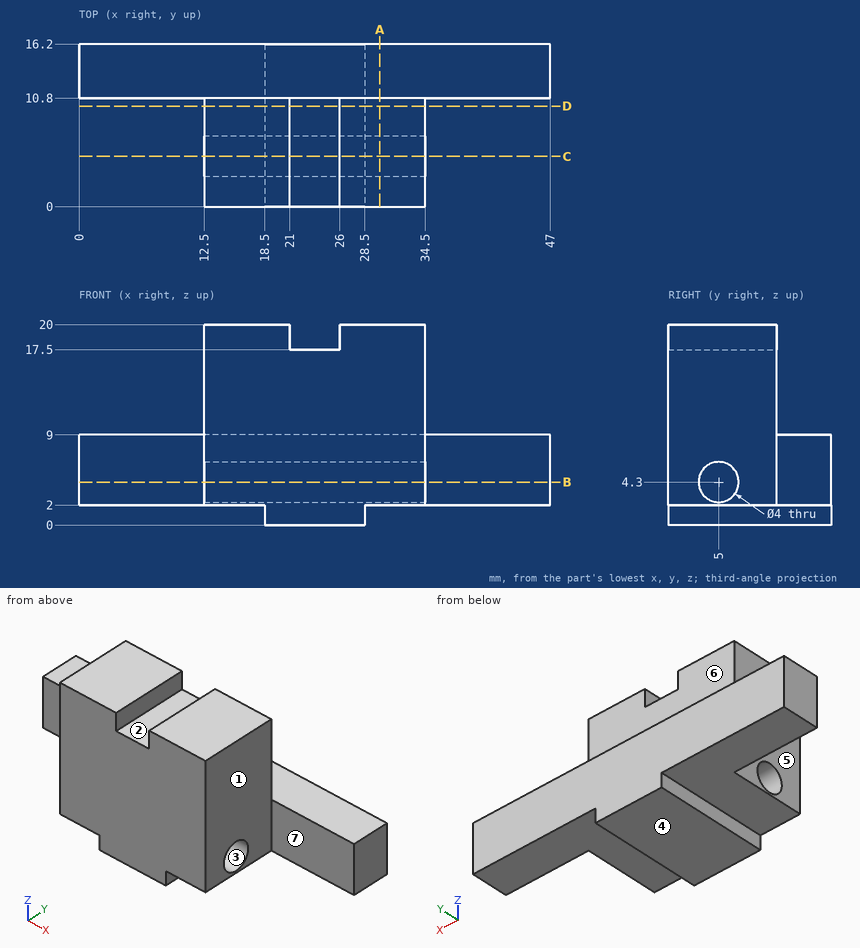
The figure shows three views and two pictorial views of one solid part (mm, origin at its lowest corner). Answer the questions. A direction names the side the tool comes from. Round coordinates to 2 decimals unless told otherwise and drop trailing zeros. Loops run counter-clockwise (first coordinate to the right, second up) from the corner with the lowest first, then second, coordinate; pieces in that order, holes last. Notation, with made-up numbers: M 21,13 L 33,13 A28 cw 33,38 Z; hole C 37.5,-25 d9. An arc over 180 degrees is marked long. Write each question's results on one line, items separated by ' | '. Start each with the question number.
1) Determine the mould class of the marked faces 1, 2, 3 and 4 for opening direction Z: pulls with the +Z half, pulls with the -Z half, needs draft (parallel to the pull), parting line crosses it, or undercut.
2) Find section B-B on z = 4.3. Write down the section's boundary in (x, y).
3) Find section A-A on x = 30. Write down the section's boundary in (y, z).
4) Straight lines are drawn through the part: probe 1 along Z at (x, y) = (28, 5); probe 2 along Z at (x, y) = (17.25, 5); probe 3 along Z at (x, y) = (31.5, 9.5). For each, find the intervals that lie inside material, in ascending order.
5) Find section D-D on y = 10. Write down the section's boundary in (x, z).
6) Which of the six approach directions +Z, -Z, +X, -X, +Y, -Y give full straight-line access (tool end or side, diameter ignored) to the marked faces 5, 6 and 7?
7) Each of these flat-tipped pins is pushed along its axis until it touches: pin 1 (2.5 mm diameter, centred on x = 22.5, y = 5.5, fed in from +Z); pin 2 (6 mm diameter, centred on y = 4.5, z = 5, fed in from +X); pin 3 (5 mm diameter, centred on x = 36, y = 6.5, fed in from -Z). Where does it stop, or does it pass through?
8) Find section C-C on y = 5. Write down the section's boundary in (x, z).
Final values:
1) face 1: needs draft | face 2: pulls with the +Z half | face 3: undercut | face 4: pulls with the -Z half
2) outline: M 0,10.8 L 12.5,10.8 L 12.5,7 L 34.5,7 L 34.5,10.8 L 47,10.8 L 47,16.2 L 0,16.2 Z; M 12.5,0 L 34.5,0 L 34.5,3 L 12.5,3 Z
3) outline: M 0,2 L 16.2,2 L 16.2,9 L 10.8,9 L 10.8,20 L 0,20 Z; hole C 5,4.3 d4
4) probe 1: 0 to 2.3, 6.3 to 20 | probe 2: 2 to 2.3, 6.3 to 20 | probe 3: 2 to 20
5) outline: M 12.5,2 L 18.5,2 L 18.5,0 L 28.5,0 L 28.5,2 L 34.5,2 L 34.5,20 L 26,20 L 26,17.5 L 21,17.5 L 21,20 L 12.5,20 Z
6) face 5: +Z, -Z, -X, -Y | face 6: +Z, +X, -X, +Y | face 7: +Z, -Z, +X, -Y
7) pin 1: z = 17.5 | pin 2: x = 34.5 | pin 3: z = 2
8) outline: M 12.5,2 L 18.5,2 L 18.5,0 L 28.5,0 L 28.5,2 L 34.5,2 L 34.5,2.3 L 12.5,2.3 Z; M 12.5,6.3 L 34.5,6.3 L 34.5,20 L 26,20 L 26,17.5 L 21,17.5 L 21,20 L 12.5,20 Z
